Here's how the part is built. I have some questions about the finished solid (model axes, mm). Round coordinates to 2 decimals unless told otherwise and drop trailing zeros. Write each loop counter-clockwise with the first axis right and the second up, starting at its lowest first coordinate (ties: lowest second). Pieces come first, ordered by that corner, then holes. Notation, with made-up numbers: M 3,-27 L 13,-27 A7 ccw 13,-20 Z; hole C -28.75,52 d2. An arc over 180 degrees is marked long. Use a Markdown table: item, result. Add a question column.
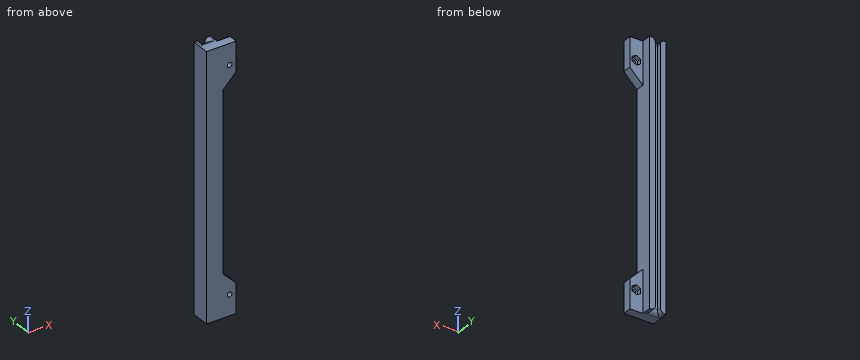
```python
from build123d import *

# Parameters (mm, degrees)
PAD_DEPTH       = 178
SKETCH001_R     = 1.6
POCKET_DEPTH    = 12.551
POCKET002_DEPTH = 5
FILLET_R        = 3


with BuildPart() as part:
    # Sketch → Pad (new body)
    with BuildSketch(Plane.XY):
        Polygon((-5.6, 0), (14.4, 0), (14.4, 5.95), (5.6, 5.95), (5.6, 12.55), (1.65, 12.55), (1.65, 9.8), (-1.65, 9.8), (-1.65, 12.55), (-5.6, 12.55), align=None)
    extrude(amount=-PAD_DEPTH)

    # Sketch001 (on Face6 of Pad) → Pocket (cut, through all)
    with BuildSketch(Plane.XZ):
        with Locations((10, -164)):
            Circle(SKETCH001_R)
        with Locations((10, -14)):
            Circle(SKETCH001_R)
        Polygon((14.4, -158), (5.6, -149.2), (5.6, -28.8), (14.4, -20), align=None)
    extrude(amount=-POCKET_DEPTH, mode=Mode.SUBTRACT)

    # Sketch003 (on DatumPlane) → Pocket002 (cut)
    with BuildSketch(Plane(origin=(0, 3, 0), x_dir=(-1, 0, 0), z_dir=(0, 1, 0))):
        Polygon((-7.2, -15.616581), (-7.2, -12.383419), (-10, -10.766838), (-12.8, -12.383419), (-12.8, -15.616581), (-10, -17.233162), align=None)
        Polygon((-7.2, -165.616581), (-7.2, -162.383419), (-10, -160.766838), (-12.8, -162.383419), (-12.8, -165.616581), (-10, -167.233162), align=None)
    extrude(amount=POCKET002_DEPTH, mode=Mode.SUBTRACT)

    # Fillet
    fillet_edges = [part.edges().sort_by_distance(p)[0] for p in [
        (-1.65, 11.175, 0),
        (0, 9.8, 0),
        (1.65, 11.175, 0),
        (0, 9.8, -178),
        (-1.65, 11.175, -178),
        (1.65, 11.175, -178),
    ]]
    fillet(fillet_edges, radius=FILLET_R)


solid = part.part
```
Item 1: Imagine slicing it at B-B on z = -141. List the corners of the cut face in (x, y) for me, plus the area to 3 significant figures.
Item 2: For pin 1 Ø1 at (x, z) = (-0.5, -55.5) entering from +Y; pin 2 Ø0.8 at (y, z) = (10.5, -120) entering from +X; pin 3 Ø1.7 at (x, z) = (10, -15) entering from +Y, each with a flat end and sliding along its axis, tell me the tip position at first contact or that it passes through.
Item 3: I need wall thicknesses on probe 1 along X at (y, z) = (1.95, -164); probe 2 along Z at (x, y) = (10.25, 5.75); probe 3 along Z at (x, y) = (10, 1.3). Which ranges of each line are inside material? Lowest first, please. Write a range as from..to.
Item 4: Imagine slicing it at A-A on z = -14. List the corners of the cut face in (x, y) for me.
The answers:
| question | item | result |
|---|---|---|
| 1 | outline | M -5.6,0 L 5.6,0 L 5.6,12.55 L 1.65,12.55 L 1.65,9.8 L -1.65,9.8 L -1.65,12.55 L -5.6,12.55 Z |
| 1 | area | 131 mm² |
| 2 | pin 1 | y = 9.8 |
| 2 | pin 2 | x = 5.6 |
| 2 | pin 3 | y = 3 |
| 3 | probe 1 | -5.6..8.4, 11.6..14.4 |
| 3 | probe 2 | -178..-167.09, -160.91..-153.85, -24.15..-17.09, -10.91..0 |
| 3 | probe 3 | -178..-165.6, -162.4..-153.6, -24.4..-15.6, -12.4..0 |
| 4 | outline | M -5.6,0 L 8.4,0 L 8.4,3 L 7.2,3 L 7.2,5.95 L 5.6,5.95 L 5.6,12.55 L 1.65,12.55 L 1.65,9.8 L -1.65,9.8 L -1.65,12.55 L -5.6,12.55 Z; M 11.6,0 L 14.4,0 L 14.4,5.95 L 12.8,5.95 L 12.8,3 L 11.6,3 Z |
